from build123d import *

# Parameters (mm, degrees)
SKETCH1_R           = 27
SKETCH1_R_2         = 2.8
BOSS_EXTRUDE2_DEPTH = 4
SKETCH2_R           = 27
SKETCH2_R_2         = 2.8
SKETCH2_R_3         = 1.5
BOSS_EXTRUDE3_DEPTH = 5
SKETCH3_R           = 3
BOSS_EXTRUDE4_DEPTH = 25
SKETCH4_R           = 12.2
SKETCH4_R_2         = 7.64
BOSS_EXTRUDE5_DEPTH = 3
SKETCH5_R           = 12.2
SKETCH5_R_2         = 7.64
CUT_EXTRUDE1_DEPTH  = 3


with BuildPart() as part:
    # Sketch1 → Boss-Extrude2 (new body)
    with BuildSketch(Plane(origin=(0, 0, 0), x_dir=(0, 0, -1), z_dir=(1, 0, 0))):
        Circle(SKETCH1_R)
        Circle(SKETCH1_R_2, mode=Mode.SUBTRACT)
    extrude(amount=BOSS_EXTRUDE2_DEPTH)

    # Sketch2 → Boss-Extrude3 (add)
    with BuildSketch(Plane(origin=(4, 0, 0), x_dir=(0, 0, -1), z_dir=(1, 0, 0))):
        Circle(SKETCH2_R)
        Circle(SKETCH2_R_2, mode=Mode.SUBTRACT)
        Circle(SKETCH2_R_2)
        Circle(SKETCH2_R_3, mode=Mode.SUBTRACT)
    extrude(amount=BOSS_EXTRUDE3_DEPTH)

    # Sketch3 → Boss-Extrude4 (add)
    with BuildSketch(Plane(origin=(9, 0, 0), x_dir=(0, 0, -1), z_dir=(1, 0, 0))):
        with Locations((0, 20)):
            Circle(SKETCH3_R)
        with Locations((17.320508076, -10)):
            Circle(SKETCH3_R)
        with Locations((-17.320508076, -10)):
            Circle(SKETCH3_R)
    extrude(amount=BOSS_EXTRUDE4_DEPTH)

    # Sketch4 → Boss-Extrude5 (add)
    with BuildSketch(Plane(origin=(9, 0, 0), x_dir=(0, 0, -1), z_dir=(1, 0, 0))):
        Circle(SKETCH4_R)
        Circle(SKETCH4_R_2, mode=Mode.SUBTRACT)
    extrude(amount=BOSS_EXTRUDE5_DEPTH)

    # Sketch5 → Cut-Extrude1 (cut)
    with BuildSketch(Plane(origin=(12, 0, 0), x_dir=(0, 0, -1), z_dir=(1, 0, 0))):
        Circle(SKETCH5_R)
        Circle(SKETCH5_R_2, mode=Mode.SUBTRACT)
    extrude(amount=-CUT_EXTRUDE1_DEPTH, mode=Mode.SUBTRACT)


solid = part.part
The listing builds one solid part. Answer for the finished solid, in the listing's coordinates (mm). A direction names the side the tool comes from. Give positions to 0.01 mm unless a question says otherwise; leave off trailing zeros. Write each loop counter-clockwise with the first axis right and the second up, starting at its lowest first coordinate (ties: lowest second). Pieces come first, ordered by that corner, then holes.
1) A tool of negligible diameter and unlimited length cuts with its end or side. For faces 1 (the face through (9, 0, -6)), 2 (the face through (34, -10, 17)), 3 (the face through (2, 0.1, 2.8)), from which of +Z, -Z, +X, -X, +Y, -Y can it reach the whole face along a straight path? Write none if from no direction.
2) Given P1, Ø8, axis at x = 12, y = 21, coming from the -Z side; P2, Ø3, axis at y = 1.5, z = 19, coming from the +X side; P3, Ø12, axis at x = 10.5, y = 8, coming from the -Z side, each flat-ended and moving along its own axis, determine where each tip first touches the part or whether it passes through.
3) For a pull along Z with two mould halves and no side action, classify faces 4 (the face through (34, 20, 0)), 5 (the face through (21.32, 17.07, 0.65)), 6 (the face through (21.325, -7.026, -16.93)) as pulls with the +Z half, pulls with the -Z half, needs draft (parallel to the pull), parting line crosses it, or undercut.
4) Find the intervals of material crossed by L1, parallel to Y at x = 6.15, z = 0; L2, parallel to Y at x = 1.7, z = 0; L3, parallel to X at y = 11.5, z = -14.5, in increasing order.
5) Section B-B (z = 0) is taken. Write down the section's boundary in (x, y), and give its area (3 significant figures).
6) Section C-C (x = 19) is taken. Write down the section's boundary in (y, z), and give its area (3 significant figures).
7) Section D-D (y = -11.5) is taken. Write down the section's boundary in (x, z).
8) Section A-A (y = 0) is taken. Write down the section's boundary in (x, z), and give its area (3 significant figures).
Response:
1. face 1: +X
1. face 2: +Z, -Z, +X, +Y, -Y
1. face 3: -X
2. P1: stops at z = -19.8
2. P2: stops at x = 9
2. P3: stops at z = -26.91
3. face 4: needs draft
3. face 5: parting line crosses it
3. face 6: undercut
4. L1: y = -27 to -1.5, 1.5 to 27
4. L2: y = -27 to -2.8, 2.8 to 27
4. L3: x = 0 to 9
5. outline: (0, -27) - (9, -27) - (9, -1.5) - (4, -1.5) - (4, -2.8) - (0, -2.8) - close; (0, 2.8) - (4, 2.8) - (4, 1.5) - (9, 1.5) - (9, 17) - (34, 17) - (34, 23) - (9, 23) - (9, 27) - (0, 27) - close
5. area: 599 mm2
6. outline: circle Ø6 at (-10, -17.32); circle Ø6 at (-10, 17.32); circle Ø6 at (20, 0)
6. area: 84.8 mm2
7. outline: (0, -24.43) - (9, -24.43) - (9, -19.92) - (34, -19.92) - (34, -14.72) - (9, -14.72) - (9, 14.72) - (34, 14.72) - (34, 19.92) - (9, 19.92) - (9, 24.43) - (0, 24.43) - close
8. outline: (0, -27) - (9, -27) - (9, -1.5) - (4, -1.5) - (4, -2.8) - (0, -2.8) - close; (0, 2.8) - (4, 2.8) - (4, 1.5) - (9, 1.5) - (9, 27) - (0, 27) - close
8. area: 449 mm2
